Verification items for the finished model (mm, model axes). A direction names the side the tool comes from. Coordinates: 2 decimals unless noted, no trailing zeros. Order: outer loops, then holes, each group sorted by start corner. A loop starts at its lowest first (then second) coordinate and runs counter-clockwise, first axis right, second up. Notation, with made-up numbers: (43, 30) -> (82, 30) arc R16 ccw to (82, 45) -> close; hole circle Ø10 at (-28, 8.5). An arc over 180 degrees is marked (long way). Answer as CSV lines item,"result".
```python
from build123d import *

# Parameters (mm, degrees)
SKETCH1_R           = 38.1
BOSS_EXTRUDE1_DEPTH = 1.1811
SKETCH2_R           = 36.5125
BOSS_EXTRUDE2_DEPTH = 1.1811
SKETCH3_R           = 3.175
CUT_EXTRUDE1_DEPTH  = 54.933292027


with BuildPart() as part:
    # Sketch1 → Boss-Extrude1 (new body)
    with BuildSketch(Plane.YZ):
        with Locations(Location((0, 0, 0), (0, 0, 270))):
            Circle(SKETCH1_R)
    extrude(amount=BOSS_EXTRUDE1_DEPTH)

    # Sketch2 → Boss-Extrude2 (add)
    with BuildSketch(Plane.YZ.offset(1.1811)):
        with Locations(Location((0, 0, 0), (0, 0, 270))):
            Circle(SKETCH2_R)
    extrude(amount=BOSS_EXTRUDE2_DEPTH)

    # Sketch3 → Cut-Extrude1 (cut, through all)
    with BuildSketch(Plane(origin=(0, 0, 0), x_dir=(0, -1, 0), z_dir=(-1, 0, 0))):
        with Locations(Location((19.05, 0, 0), (0, 0, 90))):
            Circle(SKETCH3_R)
        with Locations(Location((-19.05, 0, 0), (0, 0, 90))):
            Circle(SKETCH3_R)
    extrude(amount=-CUT_EXTRUDE1_DEPTH, mode=Mode.SUBTRACT)


solid = part.part
```
Item 1: Section check D-D, the plane y = 11. Record the boundary of the cut face in (x, z).
Answer list:
outline,"(0, -36.48) -> (1.18, -36.48) -> (1.18, -34.82) -> (2.36, -34.82) -> (2.36, 34.82) -> (1.18, 34.82) -> (1.18, 36.48) -> (0, 36.48) -> close"
Item 2: Section check A-A, the plane z = 0. Record the boundary of the cut face in (x, y) (1 decimal).
Answer list:
outline,"(0, -38.1) -> (1.2, -38.1) -> (1.2, -36.5) -> (2.4, -36.5) -> (2.4, -22.2) -> (0, -22.2) -> close; (0, -15.9) -> (2.4, -15.9) -> (2.4, 15.9) -> (0, 15.9) -> close; (0, 22.2) -> (2.4, 22.2) -> (2.4, 36.5) -> (1.2, 36.5) -> (1.2, 38.1) -> (0, 38.1) -> close"
Item 3: Thickness scan on line 1 (Y direction, x = 1.4, z = 0) (1 decimal); line 2 (Y direction, x = 1.75, z = -2); line 3 (Z direction, x = 1.7, y = 18.5). Record the ranges inside material, lowest first.
Answer list:
line 1,"-36.5 to -22.2, -15.9 to 15.9, 22.2 to 36.5"
line 2,"-36.46 to -21.52, -16.58 to 16.58, 21.52 to 36.46"
line 3,"-31.48 to -3.13, 3.13 to 31.48"
Item 4: Tool access check on faces 1 (the cylindrical face through (1.16, 15.95, -0.69)), 2 (the flat face through (1.181, -31, -20)). Record the directions out of +Z, -Z, +X, -X, +Y, -Y that give a thin tool (end or side, any length) a straight path to the whole face; none if there is none.
Answer list:
face 1,"+X, -X"
face 2,"+X"
Item 5: Release check for a two-part mould opening along Z. For faces 3 (the cylindrical face through (1.16, -18.1, 3.03)), 4 (the cylindrical face through (1.763, 10.967, -34.826)), 5 (the flat face through (0, 1, 1)) record: +Z half, -Z half, draft (parallel to the pull), parting line (faces both ways), or undercut.
Answer list:
face 3,"undercut"
face 4,"parting line"
face 5,"draft"
Item 6: Section check C-C, the plane y = -19.05. Record the boundary of the cut face in (x, z) (3 decimals).
Answer list:
outline,"(0, -32.996) -> (1.181, -32.996) -> (1.181, -31.149) -> (2.362, -31.149) -> (2.362, -3.175) -> (0, -3.175) -> close; (0, 3.175) -> (2.362, 3.175) -> (2.362, 31.149) -> (1.181, 31.149) -> (1.181, 32.996) -> (0, 32.996) -> close"
Item 7: Section check B-B, the plane x = 1.9. Count the separate pieces of the cut face and the enclosed holes in it, plus the area to 3 significant figures.
Answer list:
separate pieces,"1"
enclosed holes,"2"
area,"4,120 mm2"
Item 8: Depth check by flat-ended pin: pin 1 Ø3 at (y, z) = (19, 16.5) entering from -X. Enter the tip coordinate at first touch or a pass-through.
Answer list:
pin 1,"x = 0"
